CAD build for the part. Positions are in the model's coordinates, mm. Round coordinates to 2 decimals unless told otherwise and drop trailing zeros. Loops run counter-clockwise (first coordinate to the right, second up) from the corner with the lowest first, then second, coordinate; pieces in that order, holes last.
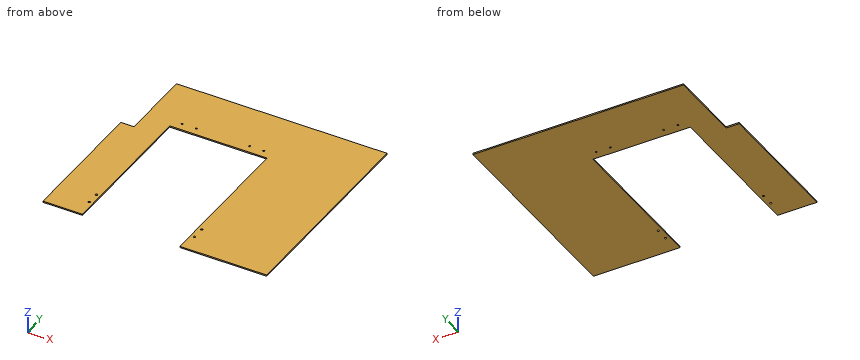
from build123d import *

# Parameters (mm, degrees)
SKETCH1_W           = 539.75
SKETCH1_H           = 508
BOSS_EXTRUDE1_DEPTH = 3.175
SKETCH2_R           = 2.54
SKETCH2_R_2         = 3.175
SKETCH2_W           = 234.95
SKETCH2_H           = 368.3
CUT_EXTRUDE1_DEPTH  = 44.45
SKETCH4_R           = 2.159
CUT_EXTRUDE3_DEPTH  = 742.218013222
CUT_EXTRUDE4_DEPTH  = 742.218013222


with BuildPart() as part:
    # Sketch1 → Boss-Extrude1 (new body)
    with BuildSketch(Plane.XY):
        with Locations((269.875, 254)):
            Rectangle(SKETCH1_W, SKETCH1_H)
    extrude(amount=BOSS_EXTRUDE1_DEPTH)

    # Sketch2 → Cut-Extrude1 (cut)
    with BuildSketch(Plane(origin=(0, 0, 0), x_dir=(-1, 0, 0), z_dir=(0, 0, -1))):
        with Locations((-339.725, 45.085)):
            Circle(SKETCH2_R)
        with Locations((-85.725, 45.085)):
            Circle(SKETCH2_R)
        with Locations((-15.24, 365.76)):
            Circle(SKETCH2_R_2)
        with Locations((-339.725, 75.565)):
            Circle(SKETCH2_R)
        with Locations((-85.725, 75.565)):
            Circle(SKETCH2_R)
        with Locations((-212.725, 184.15)):
            Rectangle(SKETCH2_W, SKETCH2_H)
    extrude(amount=-CUT_EXTRUDE1_DEPTH, mode=Mode.SUBTRACT)

    # Sketch4 → Cut-Extrude3 (cut, through all)
    with BuildSketch(Plane(origin=(0, 0, 0), x_dir=(-1, 0, 0), z_dir=(0, 0, -1))):
        with Locations((-311.1754, 387.604)):
            Circle(SKETCH4_R)
        with Locations((-277.1394, 387.604)):
            Circle(SKETCH4_R)
        with Locations((-148.3614, 387.604)):
            Circle(SKETCH4_R)
        with Locations((-114.3254, 387.604)):
            Circle(SKETCH4_R)
    extrude(amount=-CUT_EXTRUDE3_DEPTH, mode=Mode.SUBTRACT)

    # Sketch5 → Cut-Extrude4 (cut, through all)
    with BuildSketch(Plane.XY.offset(3.175)):
        Polygon((0, 403.06625), (0, 328.45375), (31.75, 328.45375), (31.75, 403.06625), (31.75, 508), (0, 508), align=None)
    extrude(amount=-CUT_EXTRUDE4_DEPTH, mode=Mode.SUBTRACT)


solid = part.part
Item 1: Cut at C-C (x = 182). List the corners of the cut face in (y, z) (3 decimals).
Verdict:
outline: (368.3, 0) - (508, 0) - (508, 3.175) - (368.3, 3.175) - close
Item 2: Cut at D-D (y = 413.5). List the corners of the cut face in (x, z) (3 decimals), plus the area to 3 significant figures.
Verdict:
outline: (31.75, 0) - (539.75, 0) - (539.75, 3.175) - (31.75, 3.175) - close
area: 1,610 mm2
Item 3: Wall check: L1, parallel to X at y = 29, z = 2.1; L2, parallel to X at y = 338, z = 2.7; L3, parallel to Y at x = 211, z = 2.65. Give the ranges that are in metal, low to high.
Verdict:
L1: x = 0 to 95.25, 330.2 to 539.75
L2: x = 31.75 to 95.25, 330.2 to 539.75
L3: y = 368.3 to 508
Item 4: Cut at A-A (y = 94). List the corners of the cut face in (x, z) (3 decimals), plus the area to 3 significant figures.
Verdict:
outline: (0, 0) - (95.25, 0) - (95.25, 3.175) - (0, 3.175) - close; (330.2, 0) - (539.75, 0) - (539.75, 3.175) - (330.2, 3.175) - close
area: 968 mm2
Item 5: Cut at B-B (z = 1.3). State how many separate pieces and enclosed holes the cut face has, plus the area to 3 significant figures.
Verdict:
separate pieces: 1
enclosed holes: 8
area: 182,000 mm2
Item 6: Flat gauge pins, fed straight in: P1, Ø5.5, axis at x = 311.18, y = 387.6, coming from the -Z side; P2, Ø1, axis at x = 9.5, z = 1, coming from the +Y side; P3, Ø1, axis at y = 424.5, z = 2.5, coming from the -X side. Where does each tip first touch, or does it go through?
Verdict:
P1: stops at z = 0
P2: stops at y = 328.45
P3: stops at x = 31.75
